Source: CAD feature listing. Evaluate the final solid. Frame: model axes, mm. Round coordinates to 2 decimals unless told otherwise and drop trailing zeros. Loops run counter-clockwise (first coordinate to the right, second up) from the corner with the lowest first, then second, coordinate; pieces in that order, holes last. Notation, with made-up numbers: M 16.5,82.5 L 56.5,82.5 A24 ccw 56.5,95.5 Z; hole C 10.5,76 d9. An arc over 180 degrees is marked long. Write each question's results on one line, items separated by ' | '. Start each with the question number.
1. Ray query, line 1 (X direction, y = 2.5, z = 3.5); line 2 (X direction, y = 1.75, z = 0.5). Return the intervals inside material, ascending.
2. Contact query for a flat-ended pin moving along its axis: pin 1 Ø1 at (y, z) = (-1, 4.5) entering from -X. Output: stop coordinate, or through.
3. Section A-A on z = -0.5. Output: boundary loops of the cut face in (x, y) (3 decimals).
4. Section C-C on y = 2. Output: boundary loops of the cut face in (x, z), and give its area (3 significant figures).
5. Section B-B on y = -1. Output: boundary loops of the cut face in (x, z).
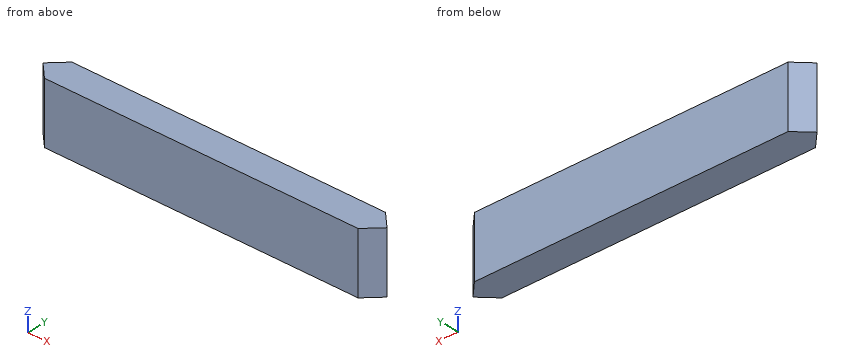
from build123d import *

# Parameters (mm, degrees)
F0_W             = 6.35
F0_H             = 12.7
F1_DEPTH         = 35.92068
F3_DEPTH         = 6.351
F3_DEPTH_BACK    = 6.351
F3_COPIES2_COUNT = 2


# Not quite as in the source:
# - a pattern or mirror of a feature is missing from the dataset's text; its kind, count and spacing are read off the source's solid


with BuildPart() as f1:
    # F0 (on Right) → F1 (new body, symmetric)
    with BuildSketch(Plane.YZ):
        Rectangle(F0_W, F0_H)
    extrude(amount=F1_DEPTH, both=True)

    # F2 (on Top) → F3 (cut, two sides)
    with BuildSketch(Plane.XY) as f3_sk:
        Polygon((-35.92068, 3.175), (-35.92068, 0), (-32.74568, 3.175), align=None)
    f3 = extrude(amount=-F3_DEPTH, mode=Mode.SUBTRACT) + extrude(f3_sk.sketch, amount=F3_DEPTH_BACK, mode=Mode.SUBTRACT)

    # F3_copies: F3 across plane
    add(f3.mirror(Plane(origin=(0, 0, 0), x_dir=(0, 0, -1), z_dir=(0, -1, 0))), mode=Mode.SUBTRACT)

    # F3_copies1: F3 across plane
    add(f3.mirror(Plane(origin=(0, 0, 0), x_dir=(0, 0, 1), z_dir=(1, 0, 0))), mode=Mode.SUBTRACT)

    # F3_copies2: F3 ×2 about axis
    f3_copies2_axis = Axis((0, 0, 0), (0, 0, 1))
    for i in range(1, F3_COPIES2_COUNT):
        add(f3.rotate(f3_copies2_axis, i * 360 / F3_COPIES2_COUNT), mode=Mode.SUBTRACT)


solid = f1.part
Taken from the geometry:
1) line 1: -33.42 to 33.42 | line 2: -34.17 to 34.17
2) pin 1: x = -35.42
3) outline: M -35.921,0 L -32.746,-3.175 L 32.746,-3.175 L 35.921,0 L 32.746,3.175 L -32.746,3.175 Z
4) outline: M -33.92,-6.35 L 33.92,-6.35 L 33.92,6.35 L -33.92,6.35 Z | area: 862 mm^2
5) outline: M -34.92,-6.35 L 34.92,-6.35 L 34.92,6.35 L -34.92,6.35 Z
